from build123d import *

# Parameters (mm, degrees)
BOSS_EXTRU_1_DEPTH      = 8
ENL_V_MAT_EXTRU_1_REACH = 183.904
ESQUISSE2_R             = 2.5
BOSS_EXTRU_2_DEPTH      = 2.5
BOSS_EXTRU_2_DEPTH_BACK = 2.5
ESQUISSE4_R             = 2.5
ENL_V_MAT_EXTRU_2_DEPTH = 8


with BuildPart() as part:
    # Esquisse1 → Boss.-Extru.1 (new body)
    with BuildSketch(Plane.XY):
        Polygon((-29, -25), (-29, -10), (-4, -10), (-4, -25), (4, -25), (4, -10), (29, -10), (29, -25), (90, -25), (90, 25), (-90, 25), (-90, -25), align=None)
    extrude(amount=BOSS_EXTRU_1_DEPTH)

    # Enlèv. mat.-Extru.1: up to this face of the body (flat: up to its plane)
    enl_v_mat_extru_1_end = Plane(part.part.faces().sort_by_distance((90, 0, 4))[0])
    # Esquisse2 → Enlèv. mat.-Extru.1 (cut, up to the picked face)
    with BuildSketch(Plane.ZY.offset(90), mode=Mode.PRIVATE) as enl_v_mat_extru_1_sk1:
        with BuildLine():
            add(Edge.make_bspline(
                [(4, -25), (6, -25), (8, -22.5)],
                knots=[0.5, 0.5, 0.5, 1, 1, 1], degree=2))
            Line((4, -25), (8, -25))
            Line((8, -25), (8, -22.5))
        make_face()
    enl_v_mat_extru_1_tool1 = split(extrude(enl_v_mat_extru_1_sk1.sketch, amount=-ENL_V_MAT_EXTRU_1_REACH, mode=Mode.PRIVATE), bisect_by=enl_v_mat_extru_1_end, keep=Keep.BOTH, mode=Mode.PRIVATE)
    # Esquisse2 → Enlèv. mat.-Extru.1 (cut, up to the picked face)
    with BuildSketch(Plane.ZY.offset(90), mode=Mode.PRIVATE) as enl_v_mat_extru_1_sk2:
        with BuildLine():
            add(Edge.make_bspline(
                [(0, -22.5), (2, -25), (4, -25)],
                knots=[0, 0, 0, 0.5, 0.5, 0.5], degree=2))
            Line((0, -22.5), (0, -25))
            Line((0, -25), (4, -25))
        make_face()
    enl_v_mat_extru_1_tool2 = split(extrude(enl_v_mat_extru_1_sk2.sketch, amount=-ENL_V_MAT_EXTRU_1_REACH, mode=Mode.PRIVATE), bisect_by=enl_v_mat_extru_1_end, keep=Keep.BOTH, mode=Mode.PRIVATE)
    # Esquisse2 → Enlèv. mat.-Extru.1 (cut, up to the picked face)
    with BuildSketch(Plane.ZY.offset(90), mode=Mode.PRIVATE) as enl_v_mat_extru_1_sk3:
        with Locations((4, -20)):
            Circle(ESQUISSE2_R)
    enl_v_mat_extru_1_tool3 = split(extrude(enl_v_mat_extru_1_sk3.sketch, amount=-ENL_V_MAT_EXTRU_1_REACH, mode=Mode.PRIVATE), bisect_by=enl_v_mat_extru_1_end, keep=Keep.BOTH, mode=Mode.PRIVATE)
    add(enl_v_mat_extru_1_tool1.solids().sort_by(Axis((-90, -24.25, 7), (1, 0, 0)))[0], mode=Mode.SUBTRACT)
    add(enl_v_mat_extru_1_tool2.solids().sort_by(Axis((-90, -24.25, 1), (1, 0, 0)))[0], mode=Mode.SUBTRACT)
    add(enl_v_mat_extru_1_tool3.solids().sort_by(Axis((-90, -20, 4), (1, 0, 0)))[0], mode=Mode.SUBTRACT)

    # Esquisse4 → Boss.-Extru.2 (add, two sides: drawn at the far end of the back side and taken through both)
    with BuildSketch(Plane(origin=(0, 0, 0), x_dir=(0, 0, -1), z_dir=(1, 0, 0)).offset(-BOSS_EXTRU_2_DEPTH_BACK)):
        with BuildLine():
            Line((5, 4.5), (0, 4.5))
            Line((0, 4.5), (0, -4.5))
            Line((0, -4.5), (5, -4.5))
            ThreePointArc((5, -4.5), (9.5, 0), (5, 4.5))
        make_face()
        with Locations((5, 0)):
            Circle(ESQUISSE4_R, mode=Mode.SUBTRACT)
    extrude(amount=BOSS_EXTRU_2_DEPTH + BOSS_EXTRU_2_DEPTH_BACK)

    # Esquisse6 → Enlèv. mat.-Extru.2 (cut)
    with BuildSketch(Plane.ZY.offset(4)):
        with BuildLine():
            add(Edge.make_bspline(
                [(0, -22.5), (4, -17.5), (8, -22.5)],
                knots=[0, 0, 0, 1, 1, 1], degree=2))
            add(Edge.make_bspline(
                [(0, -22.5), (4, -27.5), (8, -22.5)],
                knots=[0, 0, 0, 1, 1, 1], degree=2))
        make_face()
    extrude(amount=-ENL_V_MAT_EXTRU_2_DEPTH, mode=Mode.SUBTRACT)


solid = part.part
Build history of the part. All positions in model axes, mm. A direction names the side the tool comes from. Round coordinates to 2 decimals unless told otherwise and drop trailing zeros. Loops run counter-clockwise (first coordinate to the right, second up) from the corner with the lowest first, then second, coordinate; pieces in that order, holes last. Notation, with made-up numbers: (74.25, 30.5) -> (96.25, 30.5) arc R26 cw to (96.25, 54.5) -> close; hole circle Ø6 at (-9.5, -33.5). An arc over 180 degrees is marked (long way). Use CSV: the item, a comma, the result in double quotes. Start each with the question number.
Q1. Mould opens along X. For faces 1 (the face through (90, 0, 4)), 2 (the face through (-29, -16, 4)), 3 (the face through (0, 4.5, -3)) say: +X half, -X half, draft (parallel to the pull), parting line (faces both ways), or undercut.
Q2. Which spindle directions (+Z, -Z, +X, -X, +Y, -Y) get a long thin tool onto all of the face, cutting with end or side? Do faces 4 (the face through (2.5, 1.06, -2.57)), 5 (the face through (0, -4.5, -2)), 6 (the face through (29, -16, 4)). Say none if no direction does.
Q3. Flat gauge pins, fed straight in: pin 1 Ø7 at (y, z) = (1.5, -4.5) entering from +X; pin 2 Ø4.5 at (y, z) = (1, -2.5) entering from -X; pin 3 Ø2 at (x, y) = (69.5, 4) entering from -Z; pin 4 Ø2.5 at (y, z) = (-20.5, 5) entering from +X. Where does each tip first touch, or does it go through?
Q4. Saw through at B-B on x = 6.5. Give the cut face in (y, z), and give its area (3 significant figures).
Q5. Saw through at A-A on y = 8. Give the cut face in (x, z).
Q6. Drill centre lines: L1, parallel to X at y = -11, z = 1; L2, parallel to Y at x = 53.5, z = 4; L3, parallel to Y at x = 1.4, z = -5. Where is each one in solid material? Low to high.
Solutions:
1,face 1,"+X half"
1,face 2,"undercut"
1,face 3,"draft"
2,face 4,"-Z, +X, +Y, -Y"
2,face 5,"-Z, +X, -X, -Y"
2,face 6,"+Z, -Z, -Y"
3,pin 1,"stops at x = 2.5"
3,pin 2,"stops at x = -2.5"
3,pin 3,"stops at z = 0"
3,pin 4,"passes through"
4,outline,"(-10, 0) -> (25, 0) -> (25, 8) -> (-10, 8) -> close"
4,area,"280 mm^2"
5,outline,"(-90, 0) -> (90, 0) -> (90, 8) -> (-90, 8) -> close"
6,L1,"x = -90 to -29, -4 to 4, 29 to 90"
6,L2,"y = -25 to -22.5, -17.5 to 25"
6,L3,"y = -4.5 to -2.5, 2.5 to 4.5"
